Read the model definition and answer for the solid it produces. Units are mm, in the model's axes. Face numbers are marked on the shaded views. A direction names the side the tool comes from. Coordinates: 2 decimals unless noted, no trailing zeros. Write each loop counter-clockwise with the first axis right and the second up, starting at its lowest first coordinate (ties: lowest second). Pieces come first, ordered by that corner, then holes.
Item 1: Section B-B (z = 14.5) is taken. Give the vertices of the cut face in (x, y).
Item 2: Section A-A (x = 58) is taken. Give the vertices of the cut face in (y, z).
Item 3: Each of these flat-tipped pins is pushed along its axis until it touches: P1, Ø0.9, axis at x = -26.5, y = -5.5, coming from the +Z side; P2, Ø0.9, axis at y = -5.5, z = 11.5, coming from the -X side; P3, Ø0.9, axis at y = 5, z = 16, coming from the +X side; P4, Ø6, axis at x = -52.5, y = 0, coming from the -Z side. Where does it stop, or does it pass through?
Item 4: Section C-C (x = -65.5) is taken. Give the vertices of the cut face in (y, z), then the cut area to 3 significant figures.
Item 5: A tool of negligible diameter and unlimited length cuts with its end or side. For the marked faces 4, 5 and 6, from which of +Z, -Z, +X, -X, +Y, -Y can it reach the whole face along a straight path? Write none if from no direction.
Item 6: Straight lines are drawn through the part: probe 1 along X at (y, z) = (2, 14); probe 2 along Y at (x, z) = (62, 3.25); probe 3 along Z at (x, y) = (13, -4.5). For each, find the intervals that lie inside material, in ascending order.
Item 7: Determine the mould class of the marked faces 1, 2 and 3 for opening direction Y: released by +Y, released by -Y, zero draft, split by the parting line, or undercut.
from build123d import *

# Parameters (mm, degrees)
F1_W         = 164.3
F1_H         = 14.4
F1_W_2       = 158.3
F1_H_2       = 8.4
F2_DEPTH     = 24
F3_T1_DEPTH  = 24
F5_DEPTH     = 4.35
F6_W         = 14.4
F6_H         = 7
F8_W         = 40
F8_H         = 4
F10_T1_DEPTH = 90.717403587
F11_W        = 124.3
F11_H        = 14.4
F12_DEPTH    = 16
F13_R        = 5


# Not quite as in the source:
# - a fillet or chamfer that OpenCascade refuses, or shapes differently, is made with other operations: its cross-section is extruded or revolved along the edge and cut away or added
# - a pattern or mirror of a feature is missing from the dataset's text; its kind, count and spacing are read off the source's solid


with BuildPart() as f2:
    # F1 (on Top) → F2 (new body)
    with BuildSketch(Plane.XY):
        Rectangle(F1_W, F1_H)
        Rectangle(F1_W_2, F1_H_2, mode=Mode.SUBTRACT)
    extrude(amount=F2_DEPTH)

    # F3: fillet of radius 2 on 4 edges, made by hand

    # F3_s2 → F3_t1 (join)
    with BuildSketch(Plane.XY):
        with BuildLine():
            ThreePointArc((79.1504, -2.1990343146), (78.5642135624, -3.6142135624), (77.1490343146, -4.2004))
            Line((77.1490343146, -4.2004), (77.1490343146, -4.4005365685))
            ThreePointArc((77.1490343146, -4.4005365685), (78.1495171573, -4.4001365685), (79.15, -4.4001365685))
            Line((79.15, -4.4001365685), (79.3501365685, -4.2))
            ThreePointArc((79.3501365685, -4.2), (79.3501365685, -3.1995171573), (79.3505365685, -2.1990343146))
            Line((79.3505365685, -2.1990343146), (79.1504, -2.1990343146))
        make_face()
        with BuildLine():
            ThreePointArc((79.1504, 2.1990343146), (78.5642135624, 3.6142135624), (77.1490343146, 4.2004))
            Line((77.1490343146, 4.2004), (77.1490343146, 4.4005365685))
            ThreePointArc((77.1490343146, 4.4005365685), (78.1495171573, 4.4001365685), (79.15, 4.4001365685))
            Line((79.15, 4.4001365685), (79.3501365685, 4.2))
            ThreePointArc((79.3501365685, 4.2), (79.3501365685, 3.1995171573), (79.3505365685, 2.1990343146))
            Line((79.3505365685, 2.1990343146), (79.1504, 2.1990343146))
        make_face()
        with BuildLine():
            ThreePointArc((-77.1490343146, -4.2004), (-78.5642135624, -3.6142135624), (-79.1504, -2.1990343146))
            Line((-79.1504, -2.1990343146), (-79.3505365685, -2.1990343146))
            ThreePointArc((-79.3505365685, -2.1990343146), (-79.3501365685, -3.1995171573), (-79.3501365685, -4.2))
            Line((-79.3501365685, -4.2), (-79.15, -4.4001365685))
            ThreePointArc((-79.15, -4.4001365685), (-78.1495171573, -4.4001365685), (-77.1490343146, -4.4005365685))
            Line((-77.1490343146, -4.4005365685), (-77.1490343146, -4.2004))
        make_face()
        with BuildLine():
            ThreePointArc((-79.1504, 2.1990343146), (-78.5642135624, 3.6142135624), (-77.1490343146, 4.2004))
            Line((-77.1490343146, 4.2004), (-77.1490343146, 4.4005365685))
            ThreePointArc((-77.1490343146, 4.4005365685), (-78.1495171573, 4.4001365685), (-79.15, 4.4001365685))
            Line((-79.15, 4.4001365685), (-79.3501365685, 4.2))
            ThreePointArc((-79.3501365685, 4.2), (-79.3501365685, 3.1995171573), (-79.3505365685, 2.1990343146))
            Line((-79.3505365685, 2.1990343146), (-79.1504, 2.1990343146))
        make_face()
    extrude(amount=F3_T1_DEPTH)

    # F4 (on Front) → F5 (join, symmetric)
    with BuildSketch(Plane.XZ):
        with BuildLine():
            ThreePointArc((79.15, 8.75), (76.8068542495, 3.0931457505), (71.15, 0.75))
            Line((71.15, 0.75), (71.15, 0))
            Line((71.15, 0), (82.15, 0))
            Line((82.15, 0), (82.15, 8.75))
            Line((82.15, 8.75), (79.15, 8.75))
        make_face()
    f5 = extrude(amount=F5_DEPTH, both=True)

    # F5_copies: F5 across plane
    add(f5.mirror(Plane(origin=(0, 0, 0), x_dir=(0, 0, -1), z_dir=(-1, 0, 0))))

    # F6 (on face) → F9 section 0
    with BuildSketch(Plane(origin=(-82.15, 0, 0), x_dir=(0, -1, 0), z_dir=(-1, 0, 0))):
        with Locations((0, 3.5)):
            Rectangle(F6_W, F6_H)
    # F8 (on offset) → F9 section 1
    with BuildSketch(Plane(origin=(-97.15, 0, 0), x_dir=(0, -1, 0), z_dir=(-1, 0, 0))):
        with Locations((0, 2)):
            Rectangle(F8_W, F8_H)
    f9 = loft()

    # F9_copies: F9 across plane
    add(f9.mirror(Plane(origin=(0, 0, 0), x_dir=(0, 0, 1), z_dir=(1, 0, 0))))

    # F10: fillet of radius 8 on 4 edges, made by hand

    # F10_s2 → F10_t1 (cut)
    with BuildSketch(Plane.XY.offset(-43.3587017935)):
        with BuildLine():
            ThreePointArc((-97.15, 2.6565192826), (-92.500848152, 9.9209405715), (-83.9570458344, 8.7420124454))
            Line((-83.9570458344, 8.7420124454), (-97.15, 20))
            Line((-97.15, 20), (-97.15, 2.6565192826))
        make_face()
        with BuildLine():
            ThreePointArc((-83.9570458344, -8.7420124454), (-92.500848152, -9.9209405715), (-97.15, -2.6565192826))
            Line((-97.15, -2.6565192826), (-97.15, -20))
            Line((-97.15, -20), (-83.9570458344, -8.7420124454))
        make_face()
        with BuildLine():
            ThreePointArc((83.9570458344, -8.7420124454), (92.500848152, -9.9209405715), (97.15, -2.6565192826))
            Line((97.15, -2.6565192826), (97.15, -20))
            Line((97.15, -20), (83.9570458344, -8.7420124454))
        make_face()
        with BuildLine():
            ThreePointArc((97.15, 2.6565192826), (92.500848152, 9.9209405715), (83.9570458344, 8.7420124454))
            Line((83.9570458344, 8.7420124454), (97.15, 20))
            Line((97.15, 20), (97.15, 2.6565192826))
        make_face()
    extrude(amount=F10_T1_DEPTH, mode=Mode.SUBTRACT)

    # F11 (on face) → F12 (cut)
    with BuildSketch(Plane.XY.offset(24)):
        Rectangle(F11_W, F11_H)
    extrude(amount=-F12_DEPTH, mode=Mode.SUBTRACT)

    # F13
    f13_edges = [f2.edges().sort_by_distance(p)[0] for p in [
        (-62.15, 5.7, 24),
        (-62.15, -5.7, 24),
        (62.15, 5.7, 24),
        (62.15, -5.7, 24),
    ]]
    fillet(f13_edges, radius=F13_R)


solid = f2.part
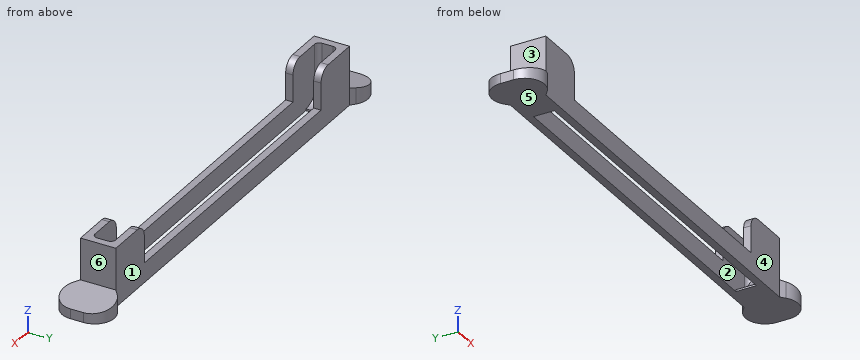
Established:
1. outline: (-82.15, -7.2) - (-62.15, -7.2) - (-62.15, -4.2) - (-77.19, -4.2) arc R2 cw to (-79.15, -2.24) - (-79.15, 2.24) arc R2 cw to (-77.19, 4.2) - (-62.15, 4.2) - (-62.15, 7.2) - (-82.15, 7.2) - close; (62.15, -7.2) - (82.15, -7.2) - (82.15, 7.2) - (62.15, 7.2) - (62.15, 4.2) - (77.19, 4.2) arc R2 cw to (79.15, 2.24) - (79.15, -2.24) arc R2 cw to (77.19, -4.2) - (62.15, -4.2) - close
2. outline: (-7.2, 0) - (-4.2, 0) - (-4.2, 8) - (-7.2, 8) - close; (4.2, 0) - (7.2, 0) - (7.2, 8) - (4.2, 8) - close
3. P1: stops at z = 8
3. P2: stops at x = -82.15
3. P3: stops at x = 82.15
3. P4: passes through
4. outline: (-7.2, 0) - (-4.2, 0) - (-4.2, 23.72) - (-7.2, 23.72) - close; (4.2, 0) - (7.2, 0) - (7.2, 23.72) - (4.2, 23.72) - close
4. area: 142 mm2
5. face 4: +Z, -Z, -Y
5. face 5: -Z, +X, -X, +Y, -Y
5. face 6: +Z, +X, +Y, -Y
6. probe 1: x = -82.15 to -79.15, 79.15 to 82.15
6. probe 2: y = -7.2 to -4.2, 4.2 to 7.2
6. probe 3: z = 0 to 8
7. face 1: released by +Y
7. face 2: undercut
7. face 3: zero draft
